Can you work these out from the drawing? Everything is in mm from the part's minimum corner. A direction names the side the tool comes from. Round coordinates to 2 decimals unless told otherwise and drop trailing zeros. Loops run counter-clockwise (first coordinate to the right, second up) from the corner with the lowest first, then second, coordinate; pieces in that order, holes last. Notation, with made-up numbers: (44.25, 55.5) - (88.25, 55.5) arc R21 ccw to (88.25, 64.5) - close; hole circle Ø4 at (3, 85). An arc over 180 degrees is marked (long way). Answer as CSV lines item,"result". Start each with the question number.
1) We'd pull the mould along Y, two halves only. Please class the marked faces 1, 2, 3 and 4: pulls with the +Y half, pulls with the -Y half, needs draft (parallel to the pull), parting line crosses it, or undercut.
2) Suppose I cut it at A-A, the plane z = 15. Write out the boundary of the cut face in (x, y).
3) Suppose I cut it at B-B, the plane x = 6. Write out the boundary of the cut face in (y, z).
4) Suppose I cut it at D-D, the plane y = 31. Write out the boundary of the cut face in (x, z), then the cut area to 3 significant figures.
5) Which directions (+Z, -Z, +X, -X, +Y, -Y) give clear straight access to the entire face, cutting with the end or side of a thin tool? Please do the marked faces 5 and 6.
6) Suppose I cut it at C-C, the plane y = 20. Write out the boundary of the cut face in (x, z), then the cut area to 3 significant figures.
7) Please list where these lines run through material, in increasing order: line 1 along Y through (x, z) = (32, 18.75); line 2 along X through (y, z) = (33, 9.25); line 3 along Y through (x, z) = (2.4, 15).
8) I'm going to push flat-ended pins straight in: pin 1 Ø9 at (y, z) = (22, 10) entering from +X; pin 2 Ø1.5 at (x, z) = (37.5, 25) entering from -Y. Where does each tip first touch, or does it pass through?
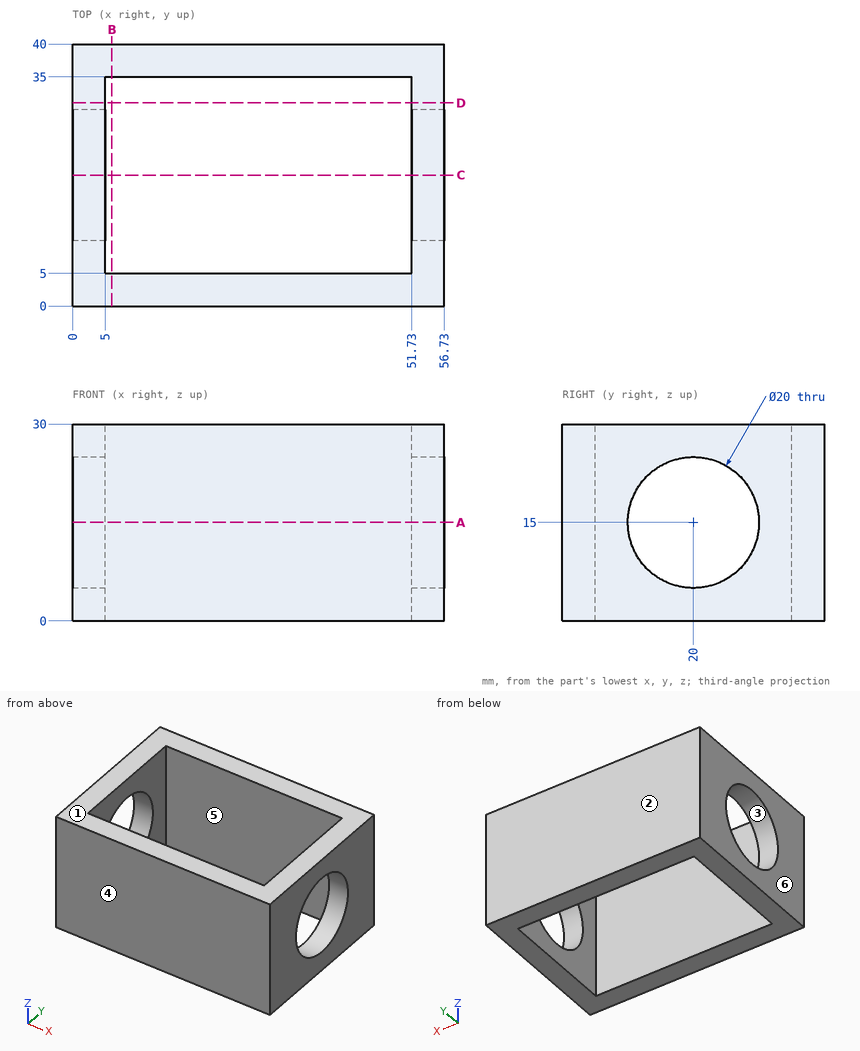
Filled sheet:
1,face 1,"needs draft"
1,face 2,"pulls with the +Y half"
1,face 3,"undercut"
1,face 4,"pulls with the -Y half"
2,outline,"(0, 0) - (56.73, 0) - (56.73, 10) - (51.73, 10) - (51.73, 5) - (5, 5) - (5, 10) - (0, 10) - close; (0, 30) - (5, 30) - (5, 35) - (51.73, 35) - (51.73, 30) - (56.73, 30) - (56.73, 40) - (0, 40) - close"
3,outline,"(0, 0) - (5, 0) - (5, 30) - (0, 30) - close; (35, 0) - (40, 0) - (40, 30) - (35, 30) - close"
4,outline,"(0, 0) - (5, 0) - (5, 30) - (0, 30) - close; (51.73, 0) - (56.73, 0) - (56.73, 30) - (51.73, 30) - close"
4,area,"300 mm²"
5,face 5,"+Z, -Z"
5,face 6,"+Z, -Z, -X, +Y, -Y"
6,outline,"(0, 0) - (5, 0) - (5, 5) - (0, 5) - close; (0, 25) - (5, 25) - (5, 30) - (0, 30) - close; (51.73, 0) - (56.73, 0) - (56.73, 5) - (51.73, 5) - close; (51.73, 25) - (56.73, 25) - (56.73, 30) - (51.73, 30) - close"
6,area,"100 mm²"
7,line 1,"0 to 5, 35 to 40"
7,line 2,"0 to 5, 51.73 to 56.73"
7,line 3,"0 to 10, 30 to 40"
8,pin 1,"through"
8,pin 2,"y = 0"
